from build123d import *

# Parameters (mm, degrees)
F0_R          = 7.1
F0_R_2        = 2.1
F1_DEPTH      = 47.7
F3_DEPTH      = 3.2
F4_R          = 3.75
F5_DEPTH      = 1
F6_W          = 8
F6_H          = 35.7
F7_DEPTH      = 25
F9_START      = -2.5
F8_R          = 5.1
F9_DEPTH      = 37.5
F10_T1_DEPTH  = 35.7
F10_T8_ANGLE  = 100.8666218277
F10_T14_ANGLE = 100.8666218277
F10_T23_DEPTH = 40.4388611997
F10_T27_ANGLE = 100.8666218277
F10_T34_ANGLE = 100.8666218277
F10_T38_DEPTH = 40.4388611997
F10_T45_DEPTH = 40.4388611997
F10_T49_ANGLE = 100.8666218277
F10_T56_DEPTH = 40.4388611997
F10_T60_ANGLE = 100.8666218277


# Not quite as in the source:
# - a fillet or chamfer that OpenCascade refuses, or shapes differently, is made with other operations: its cross-section is extruded or revolved along the edge and cut away or added


with BuildPart() as f1:
    # F0 (on Top) → F1 (new body)
    with BuildSketch(Plane.XY):
        Circle(F0_R)
        Circle(F0_R_2, mode=Mode.SUBTRACT)
    extrude(amount=F1_DEPTH)

    # F2 (on face) → F3 (cut)
    with BuildSketch(Plane(origin=(0, 0, 0), x_dir=(1, 0, 0), z_dir=(0, 0, -1))):
        Polygon((2.6088002978, -3.8114950268), (4.6052516685, 0.3535398179), (1.9964513707, 4.1650348447), (-2.6088002978, 3.8114950268), (-4.6052516685, -0.3535398179), (-1.9964513707, -4.1650348447), align=None)
    extrude(amount=-F3_DEPTH, mode=Mode.SUBTRACT)

    # F4 (on face) → F5 (cut)
    with BuildSketch(Plane.XY.offset(47.7)):
        Circle(F4_R)
    extrude(amount=-F5_DEPTH, mode=Mode.SUBTRACT)

    # F6 (on Right) → F7 (cut)
    with BuildSketch(Plane.YZ):
        with Locations((0, 23.85)):
            Rectangle(F6_W, F6_H)
    extrude(amount=-F7_DEPTH, mode=Mode.SUBTRACT)

    # F8 (on face) → F9 (cut)
    with BuildSketch(Plane(origin=(0, 0, 3.2), x_dir=(1, 0, 0), z_dir=(0, 0, -1)).offset(F9_START)):
        Circle(F8_R)
    extrude(amount=-F9_DEPTH, mode=Mode.SUBTRACT)

    # F10: fillet of radius 0.8 on 6 edges, made by hand

    # F10_s2 → F10_t1 (cut)
    with BuildSketch(Plane.XY.offset(6)):
        with BuildLine():
            ThreePointArc((-4.5985924101, 5.4095238095), (-4.831313661, 4.5239737763), (-4.0804411526, 4))
            Line((-4.0804411526, 4), (-5.8660037504, 4))
            ThreePointArc((-5.8660037504, 4), (-5.279548517, 4.747248409), (-4.5985924101, 5.4095238095))
        make_face()
        with BuildLine():
            ThreePointArc((-4.5985924101, -5.4095238095), (-4.831313661, -4.5239737763), (-4.0804411526, -4))
            Line((-4.0804411526, -4), (-5.8660037504, -4))
            ThreePointArc((-5.8660037504, -4), (-5.279548517, -4.747248409), (-4.5985924101, -5.4095238095))
        make_face()
    extrude(amount=F10_T1_DEPTH, mode=Mode.SUBTRACT)

    # F10_s3 → F10_t4 (revolve, cut)
    with BuildSketch(Plane.XZ):
        with BuildLine():
            ThreePointArc((7.1, 0.8), (6.8656854249, 0.2343145751), (6.3, 0))
            Line((6.3, 0), (7.1, 0))
            Line((7.1, 0), (7.1, 0.8))
        make_face()
    revolve(axis=Axis((0, 0, 0), (0, 0, 1)), mode=Mode.SUBTRACT)


with BuildPart() as f10_tool6:
    # F10_s7 → F10_t8 (revolve)
    with BuildSketch(Plane(origin=(0, 0, 0), x_dir=(0, 0, 1), z_dir=(0.7708837014, -0.6369759171, 0))):
        with BuildLine():
            ThreePointArc((5.2, 7.1), (5.7656854249, 6.8656854249), (6, 6.3))
            Line((6, 6.3), (6, 7.1))
            Line((6, 7.1), (5.2, 7.1))
        make_face()
    revolve(axis=Axis((0, 0, 6), (0, 0, -1)), revolution_arc=F10_T8_ANGLE)

    split(bisect_by=Plane.XZ.offset(4), keep=Keep.BOTTOM)

    split(bisect_by=Plane.XZ.offset(-4), keep=Keep.TOP)


with BuildPart() as f1_1:
    add(f1.part)

    # F10_t5: cut F10_tool6
    add(f10_tool6.part, mode=Mode.SUBTRACT)


with BuildPart() as f10_tool12:
    # F10_s13 → F10_t14 (revolve)
    with BuildSketch(Plane(origin=(0, 0, 0), x_dir=(0, 0, 1), z_dir=(0.7708837014, -0.6369759171, 0))):
        with BuildLine():
            ThreePointArc((42.5, 7.1), (41.9343145751, 6.8656854249), (41.7, 6.3))
            Line((41.7, 6.3), (41.7, 7.1))
            Line((41.7, 7.1), (42.5, 7.1))
        make_face()
    revolve(axis=Axis((0, 0, 41.7), (0, 0, -1)), revolution_arc=F10_T14_ANGLE)

    split(bisect_by=Plane.XZ.offset(4), keep=Keep.BOTTOM)

    split(bisect_by=Plane.XZ.offset(-4), keep=Keep.TOP)


with BuildPart() as f1_2:
    add(f1_1.part)

    # F10_t11: cut F10_tool12
    add(f10_tool12.part, mode=Mode.SUBTRACT)

    # F10_s17 → F10_t18 (revolve, cut)
    with BuildSketch(Plane.XZ):
        with BuildLine():
            ThreePointArc((7.1, 46.9), (6.8656854249, 47.4656854249), (6.3, 47.7))
            Line((6.3, 47.7), (7.1, 47.7))
            Line((7.1, 47.7), (7.1, 46.9))
        make_face()
    revolve(axis=Axis((0, 0, 47.7), (0, 0, 1)), mode=Mode.SUBTRACT)


with BuildPart() as f10_tool21:
    # F10_s22 → F10_t23 (new body)
    with BuildSketch(Plane.XY.offset(41.7)):
        with BuildLine():
            ThreePointArc((-4.5985924101, -5.4095238095), (-4.831313661, -4.5239737763), (-4.0804411526, -4))
            Line((-4.0804411526, -4), (-5.8660037504, -4))
            ThreePointArc((-5.8660037504, -4), (-5.279548517, -4.747248409), (-4.5985924101, -5.4095238095))
        make_face()
    extrude(amount=-F10_T23_DEPTH)

    split(bisect_by=Plane.XY.offset(6), keep=Keep.BOTTOM)


with BuildPart() as f10_tool25:
    # F10_s26 → F10_t27 (revolve)
    with BuildSketch(Plane(origin=(0, 0, 0), x_dir=(0, 0, 1), z_dir=(0.7708837014, -0.6369759171, 0))):
        with BuildLine():
            ThreePointArc((5.2, 7.1), (5.7656854249, 6.8656854249), (6, 6.3))
            Line((6, 6.3), (6, 7.1))
            Line((6, 7.1), (5.2, 7.1))
        make_face()
    revolve(axis=Axis((0, 0, 6), (0, 0, -1)), revolution_arc=F10_T27_ANGLE)

    split(bisect_by=Plane.XZ.offset(4), keep=Keep.TOP)


with BuildPart() as f10_tool21_1:
    add(f10_tool21.part)

    # F10_t29: intersect F10_tool25
    add(f10_tool25.part, mode=Mode.INTERSECT)


with BuildPart() as f1_3:
    add(f1_2.part)

    # F10_t19: cut F10_tool21
    add(f10_tool21_1.part, mode=Mode.SUBTRACT)


with BuildPart() as f10_tool32:
    # F10_s33 → F10_t34 (revolve)
    with BuildSketch(Plane(origin=(0, 0, 0), x_dir=(0, 0, 1), z_dir=(0.7708837014, -0.6369759171, 0))):
        with BuildLine():
            ThreePointArc((5.2, 7.1), (5.7656854249, 6.8656854249), (6, 6.3))
            Line((6, 6.3), (6, 7.1))
            Line((6, 7.1), (5.2, 7.1))
        make_face()
    revolve(axis=Axis((0, 0, 6), (0, 0, -1)), revolution_arc=F10_T34_ANGLE)

    split(bisect_by=Plane.XZ.offset(-4), keep=Keep.BOTTOM)


with BuildPart() as f10_tool36:
    # F10_s37 → F10_t38 (new body)
    with BuildSketch(Plane.XY.offset(41.7)):
        with BuildLine():
            ThreePointArc((-4.5985924101, 5.4095238095), (-4.831313661, 4.5239737763), (-4.0804411526, 4))
            Line((-4.0804411526, 4), (-5.8660037504, 4))
            ThreePointArc((-5.8660037504, 4), (-5.279548517, 4.747248409), (-4.5985924101, 5.4095238095))
        make_face()
    extrude(amount=-F10_T38_DEPTH)

    split(bisect_by=Plane.XY.offset(6), keep=Keep.BOTTOM)


with BuildPart() as f10_tool32_1:
    add(f10_tool32.part)

    # F10_t40: intersect F10_tool36
    add(f10_tool36.part, mode=Mode.INTERSECT)


with BuildPart() as f1_4:
    add(f1_3.part)

    # F10_t30: cut F10_tool32
    add(f10_tool32_1.part, mode=Mode.SUBTRACT)


with BuildPart() as f10_tool43:
    # F10_s44 → F10_t45 (new body)
    with BuildSketch(Plane.XY.offset(46.4388611997)):
        with BuildLine():
            ThreePointArc((-4.5985924101, -5.4095238095), (-4.831313661, -4.5239737763), (-4.0804411526, -4))
            Line((-4.0804411526, -4), (-5.8660037504, -4))
            ThreePointArc((-5.8660037504, -4), (-5.279548517, -4.747248409), (-4.5985924101, -5.4095238095))
        make_face()
    extrude(amount=-F10_T45_DEPTH)

    split(bisect_by=Plane.XY.offset(41.7), keep=Keep.TOP)


with BuildPart() as f10_tool47:
    # F10_s48 → F10_t49 (revolve)
    with BuildSketch(Plane(origin=(0, 0, 0), x_dir=(0, 0, 1), z_dir=(0.7708837014, -0.6369759171, 0))):
        with BuildLine():
            ThreePointArc((42.5, 7.1), (41.9343145751, 6.8656854249), (41.7, 6.3))
            Line((41.7, 6.3), (41.7, 7.1))
            Line((41.7, 7.1), (42.5, 7.1))
        make_face()
    revolve(axis=Axis((0, 0, 41.7), (0, 0, -1)), revolution_arc=F10_T49_ANGLE)

    split(bisect_by=Plane.XZ.offset(4), keep=Keep.TOP)


with BuildPart() as f10_tool43_1:
    add(f10_tool43.part)

    # F10_t51: intersect F10_tool47
    add(f10_tool47.part, mode=Mode.INTERSECT)


with BuildPart() as f1_5:
    add(f1_4.part)

    # F10_t41: cut F10_tool43
    add(f10_tool43_1.part, mode=Mode.SUBTRACT)


with BuildPart() as f10_tool54:
    # F10_s55 → F10_t56 (new body)
    with BuildSketch(Plane.XY.offset(46.4388611997)):
        with BuildLine():
            ThreePointArc((-4.5985924101, 5.4095238095), (-4.831313661, 4.5239737763), (-4.0804411526, 4))
            Line((-4.0804411526, 4), (-5.8660037504, 4))
            ThreePointArc((-5.8660037504, 4), (-5.279548517, 4.747248409), (-4.5985924101, 5.4095238095))
        make_face()
    extrude(amount=-F10_T56_DEPTH)

    split(bisect_by=Plane.XY.offset(41.7), keep=Keep.TOP)


with BuildPart() as f10_tool58:
    # F10_s59 → F10_t60 (revolve)
    with BuildSketch(Plane(origin=(0, 0, 0), x_dir=(0, 0, 1), z_dir=(0.7708837014, -0.6369759171, 0))):
        with BuildLine():
            ThreePointArc((42.5, 7.1), (41.9343145751, 6.8656854249), (41.7, 6.3))
            Line((41.7, 6.3), (41.7, 7.1))
            Line((41.7, 7.1), (42.5, 7.1))
        make_face()
    revolve(axis=Axis((0, 0, 41.7), (0, 0, -1)), revolution_arc=F10_T60_ANGLE)

    split(bisect_by=Plane.XZ.offset(-4), keep=Keep.BOTTOM)


with BuildPart() as f10_tool54_1:
    add(f10_tool54.part)

    # F10_t62: intersect F10_tool58
    add(f10_tool58.part, mode=Mode.INTERSECT)


with BuildPart() as f1_6:
    add(f1_5.part)

    # F10_t52: cut F10_tool54
    add(f10_tool54_1.part, mode=Mode.SUBTRACT)


solid = f1_6.part
Could you check a few things on this model? Use its own coordinates, in mm. A direction names the side the tool comes from. Round coordinates to 2 decimals unless told otherwise and drop trailing zeros. Write each loop counter-clockwise with the first axis right and the second up, starting at its lowest first coordinate (ties: lowest second). Pieces come first, ordered by that corner, then holes. Notation, with made-up numbers: (13, 4.25) - (71, 4.25) arc R22 ccw to (71, 21.25) - close; hole circle Ø3 at (-22, 10). An arc over 180 degrees is marked (long way). Use a Markdown table: item, result.
Q1. For pin 1 (2.5 mm diameter, centred on x = 1, y = 1, fed in from -Z); pin 2 (1 mm diameter, centred on y = -4.5, z = 9.5, fed in from +X); pin 3 (1.5 mm diameter, centred on y = -1, z = 30, fed in from +X), each with a flat end and sliding along its axis, tell me the tip position at first contact or that it passes through.
Output values:
| item | result |
|---|---|
| pin 1 | z = 3.2 |
| pin 2 | x = 5.87 |
| pin 3 | x = 7.1 |
Q2. Thinking about a two-plate mould opening in Y: for faces 1 (the cylindrical face through (6.772, 2.133, 23.527)), 2 (the flat face through (-3.59, -1.76, 1.58)), 3 (the flat face through (-3, 3, 0)), which applies, released by +Y, released by -Y, zero draft, split by the parting line, or undercut?
Output values:
| item | result |
|---|---|
| face 1 | split by the parting line |
| face 2 | undercut |
| face 3 | zero draft |
Q3. I want a section at A-A (x = 0). List the corners of the cut face in (y, z) for me, plus the area to 3 significant figures.
Output values:
| item | result |
|---|---|
| outline | (-7.1, 0.8) arc R0.8 ccw to (-6.3, 0) - (-4.01, 0) - (-4.01, 3.2) - (-2.1, 3.2) - (-2.1, 5.7) - (-5.1, 5.7) - (-5.1, 43.2) - (-2.1, 43.2) - (-2.1, 46.7) - (-3.75, 46.7) - (-3.75, 47.7) - (-6.3, 47.7) arc R0.8 ccw to (-7.1, 46.9) - close; (2.1, 3.2) - (4.01, 3.2) - (4.01, 0) - (6.3, 0) arc R0.8 ccw to (7.1, 0.8) - (7.1, 46.9) arc R0.8 ccw to (6.3, 47.7) - (3.75, 47.7) - (3.75, 46.7) - (2.1, 46.7) - (2.1, 43.2) - (5.1, 43.2) - (5.1, 5.7) - (2.1, 5.7) - close |
| area | 236 mm2 |
Q4. Please list where these lines run through material, in increasing order: L1, parallel to Z at x = 0.75, y = -4; L2, parallel to Z at x = -2.25, y = 0; L3, parallel to Y at x = 0, z = 4.45.
Output values:
| item | result |
|---|---|
| L1 | 3.2 to 5.7, 43.2 to 47.7 |
| L2 | 3.2 to 5.7, 43.2 to 46.7 |
| L3 | -7.1 to -2.1, 2.1 to 7.1 |
Q5. For faces 4 (the flat face through (2.2, 1.1, 43.2)), 5 (the cylindrical face through (-3.746, 0.165, 47.207)), 6 (the cylindrical face through (-4.836, 4.537, 24.111)), which set-ups out of +Z, -Z, +X, -X, +Y, -Y let a thin tool reach every point of the face, with its end or its side?
Output values:
| item | result |
|---|---|
| face 4 | none |
| face 5 | +Z |
| face 6 | -X |
Q6. I want a section at B-B (z = 16). List the corners of the cut face in (x, y) for me, plus the area to 3 significant figures.
Output values:
| item | result |
|---|---|
| outline | (-4.6, -5.41) arc R7.1 ccw (long way) to (-4.6, 5.41) arc R0.8 ccw to (-4.08, 4) - (-3.16, 4) arc R5.1 cw (long way) to (-3.16, -4) - (-4.08, -4) arc R0.8 ccw to start |
| area | 57.6 mm2 |
